Source: three-view drawing plus pictorial views. Frame: mm from the lowest corner of the part. A direction names the side the tool comes from. Give positions to 0.01 mm unless a question says otherwise; leave off trailing zeros. Order: outer loops, then holes, each group sorted by start corner. A loop starts at its lowest first (then second) coordinate and runs counter-clockwise, first axis right, second up.
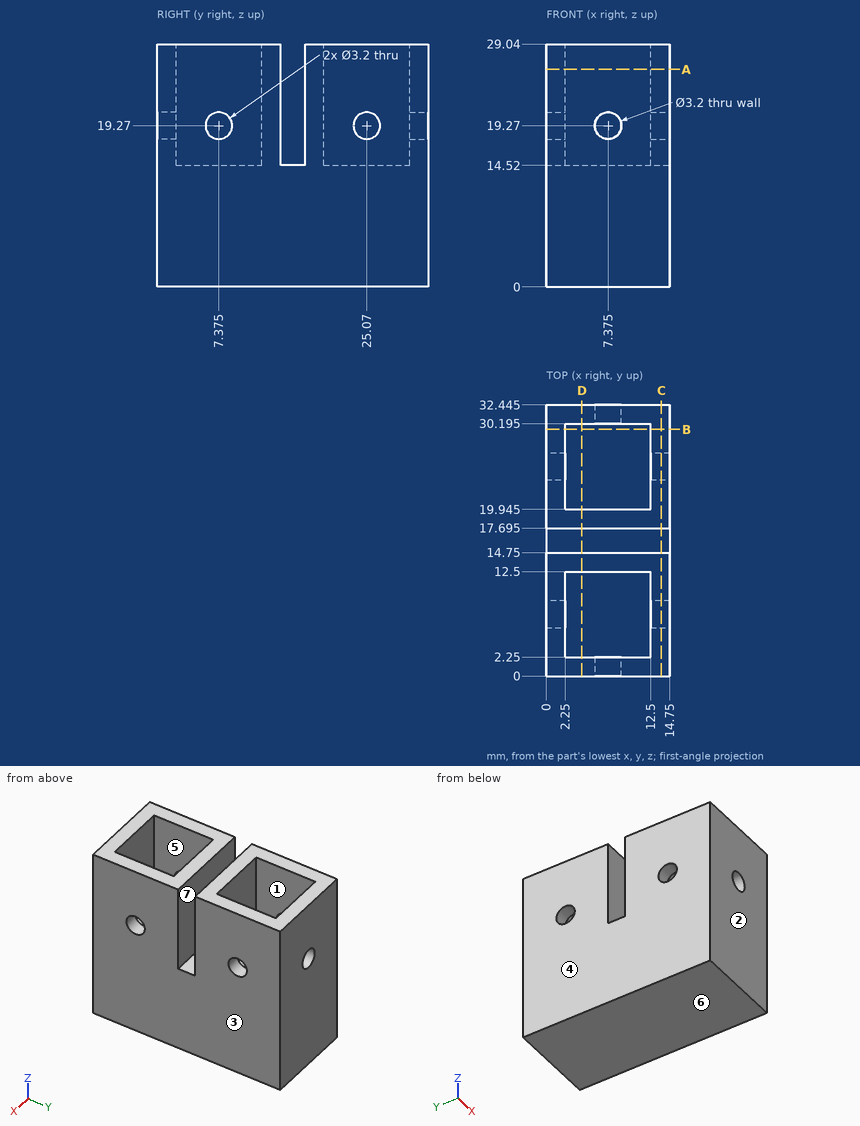
(1) Section B-B, the plane y = 29.5. Return loops of the section in (x, z).
(2) Draft query along X for the marked faces 1, 2, 3 and 4. Return one class per face: +X half, -X half, draft (parallel to the pull), parting line (faces both ways), or undercut.
(3) Pin query (flat end, axial travel): pin 1 Ø1.9 at (y, z) = (25.07, 19.27) entering from -X; pin 2 Ø1 at (x, y) = (7, 4.5) entering from +Z. Return the tip coordinate at first contact, or that it passes through.
(4) Section C-C, the plane x = 13.75. Return loops of the section in (y, z) (3 decimals), plus the area to 3 significant figures.
(5) Line query: line 1 along Y through (x, z) = (5.75, 27.5) (3 decimals); line 2 along Y through (x, z) = (6.5, 18.75) (3 decimals); line 3 along X through (y, z) = (9, 23.5). Output: solid intervals per line, ascending.
(6) Section D-D, the plane x = 4.25. Return loops of the section in (y, z) (3 decimals), plus the area to 3 significant figures.
(7) Section A-A, the plane z = 26. Return loops of the section in (x, y) (3 decimals).
(8) Access query for the marked faces 5, 6 and 7. Directions: +Z, -Z, +X, -X, +Y, -Y. A direction counts if a zero-diameter tool reaches every point of the face in a straight line with its end or side. Return the directions, or none.
Checks:
1. outline: (0, 0) - (14.75, 0) - (14.75, 29.04) - (12.5, 29.04) - (12.5, 14.52) - (2.25, 14.52) - (2.25, 29.04) - (0, 29.04) - close
2. face 1: undercut
2. face 2: draft
2. face 3: +X half
2. face 4: -X half
3. pin 1: passes through
3. pin 2: stops at z = 14.52
4. outline: (0, 0) - (32.445, 0) - (32.445, 29.04) - (17.695, 29.04) - (17.695, 14.52) - (14.75, 14.52) - (14.75, 29.04) - (0, 29.04) - close; hole circle Ø3.2 at (7.375, 19.27); hole circle Ø3.2 at (25.07, 19.27)
4. area: 883 mm2
5. line 1: y = 0 to 2.25, 12.5 to 14.75, 17.695 to 19.945, 30.195 to 32.445
5. line 2: y = 12.5 to 14.75, 17.695 to 19.945
5. line 3: x = 0 to 2.25, 12.5 to 14.75
6. outline: (0, 0) - (32.445, 0) - (32.445, 29.04) - (30.195, 29.04) - (30.195, 14.52) - (19.945, 14.52) - (19.945, 29.04) - (17.695, 29.04) - (17.695, 14.52) - (14.75, 14.52) - (14.75, 29.04) - (12.5, 29.04) - (12.5, 14.52) - (2.25, 14.52) - (2.25, 29.04) - (0, 29.04) - close
6. area: 602 mm2
7. outline: (0, 0) - (14.75, 0) - (14.75, 14.75) - (0, 14.75) - close; (0, 17.695) - (14.75, 17.695) - (14.75, 32.445) - (0, 32.445) - close; hole (2.25, 2.25) - (12.5, 2.25) - (12.5, 12.5) - (2.25, 12.5) - close; hole (2.25, 19.945) - (12.5, 19.945) - (12.5, 30.195) - (2.25, 30.195) - close
8. face 5: +Z
8. face 6: -Z, +X, -X, +Y, -Y
8. face 7: +Z, +X, -X
